```python
from build123d import *

# Parameters (mm, degrees)
SKETCH1_W           = 135.25
SKETCH1_H           = 90
BOSS_EXTRUDE1_DEPTH = 22
SKETCH4_W           = 5
SKETCH4_H           = 19
CUT_EXTRUDE1_DEPTH  = 91
SKETCH5_W           = 117.25
SKETCH5_H           = 11
CUT_EXTRUDE2_DEPTH  = 91
FILLET1_R           = 10
FILLET2_R           = 10
FILLET3_R           = 10
FILLET4_R           = 10
FILLET5_R           = 10
SKETCH6_R           = 4
CUT_EXTRUDE3_DEPTH  = 136.25


with BuildPart() as part:
    # Sketch1 → Boss-Extrude1 (new body)
    with BuildSketch(Plane(origin=(0, 0, 0), x_dir=(1, 0, 0), z_dir=(0, 1, 0))):
        Rectangle(SKETCH1_W, SKETCH1_H)
    extrude(amount=BOSS_EXTRUDE1_DEPTH)

    # Sketch4 → Cut-Extrude1 (cut, through all)
    with BuildSketch(Plane.XY.offset(45)):
        with Locations((-61.125, 9.5)):
            Rectangle(SKETCH4_W, SKETCH4_H)
        with Locations((61.125, 9.5)):
            Rectangle(SKETCH4_W, SKETCH4_H)
    extrude(amount=-CUT_EXTRUDE1_DEPTH, mode=Mode.SUBTRACT)

    # Sketch5 → Cut-Extrude2 (cut, through all)
    with BuildSketch(Plane(origin=(0, 0, -45), x_dir=(-1, 0, 0), z_dir=(0, 0, -1))):
        Rectangle(SKETCH5_W, SKETCH5_H)
    extrude(amount=-CUT_EXTRUDE2_DEPTH, mode=Mode.SUBTRACT)

    # Fillet1
    fillet1_edges = [part.edges().sort_by_distance(p)[0] for p in [
        (0, 5.5, 45),
    ]]
    fillet(fillet1_edges, radius=FILLET1_R)

    # Fillet2
    fillet2_edges = [part.edges().sort_by_distance(p)[0] for p in [
        (-65.625, 0, 45),
    ]]
    fillet(fillet2_edges, radius=FILLET2_R)

    # Fillet3
    fillet3_edges = [part.edges().sort_by_distance(p)[0] for p in [
        (65.625, 0, 45),
    ]]
    fillet(fillet3_edges, radius=FILLET3_R)

    # Fillet4
    fillet4_edges = [part.edges().sort_by_distance(p)[0] for p in [
        (-65.625, 0, -45),
    ]]
    fillet(fillet4_edges, radius=FILLET4_R)

    # Fillet5
    fillet5_edges = [part.edges().sort_by_distance(p)[0] for p in [
        (65.625, 0, -45),
    ]]
    fillet(fillet5_edges, radius=FILLET5_R)

    # Sketch6 → Cut-Extrude3 (cut, through all)
    with BuildSketch(Plane.ZY.offset(67.625)):
        with Locations((-38, 13)):
            Circle(SKETCH6_R)
    extrude(amount=-CUT_EXTRUDE3_DEPTH, mode=Mode.SUBTRACT)


solid = part.part
```
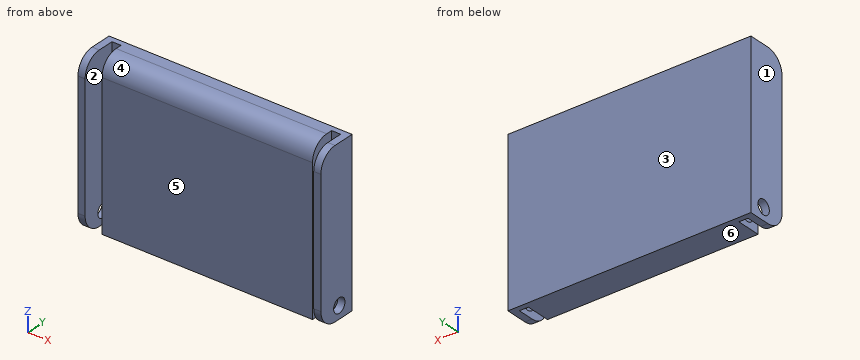
For this review, take the finished solid that the model builds, in its own axes (mm). Face numbers are marked on the shaded views. A direction names the side the tool comes from. Round coordinates to 2 decimals unless told otherwise and drop trailing zeros. Write each loop counter-clockwise with the first axis right and the second up, starting at its lowest first coordinate (ties: lowest second). Pieces come first, ordered by that corner, then holes. Notation, with made-up numbers: (11, 80.25) -> (42, 80.25) arc R23 ccw to (42, 98.25) -> close; hole circle Ø3 at (-17, 71). An arc over 180 degrees is marked (long way). Use one line per item in the form item = value.
Q1. The part is to be moulded in two halves that separate along X. For the marked faces 1, 2, 3 and 4, say which applies: released by +X, released by -X, zero draft, split by the parting line, or undercut.
Resolved:
face_1 = released by -X
face_2 = undercut
face_3 = zero draft
face_4 = undercut
Q2. Machinability: for the marked faces 5 and 6, which of the approach directions +Z, -Z, +X, -X, +Y, -Y give a long, thin tool a straight path to every point of the face, cutting with its end or side? Answer none if there is none.
Resolved:
face_5 = +Z, -Z, -Y
face_6 = -Z, +X, -X, +Y, -Y
Q3. Consider section B-B (x = 46). State the section outline as (y, z) points.
Resolved:
outline = (5.5, -45) -> (22, -45) -> (22, 45) -> (15.5, 45) arc R10 ccw to (5.5, 35) -> close; hole circle Ø8 at (13, -38)
Q4. Consider section D-D (z = -38). State the section outline as (x, y) points (3 decimals).
Resolved:
outline = (-67.625, 0.461) -> (-63.625, 0.461) -> (-63.625, 9) -> (-67.625, 9) -> close; (-67.625, 17) -> (-63.625, 17) -> (-63.625, 19) -> (-58.625, 19) -> (-58.625, 17) -> (58.625, 17) -> (58.625, 19) -> (63.625, 19) -> (63.625, 17) -> (67.625, 17) -> (67.625, 22) -> (-67.625, 22) -> close; (-58.625, 5.5) -> (58.625, 5.5) -> (58.625, 9) -> (-58.625, 9) -> close; (63.625, 0.461) -> (67.625, 0.461) -> (67.625, 9) -> (63.625, 9) -> close
Q5. Consider section C-C (y = 13). State the section outline as (x, z) points (3 decimals), then the cut area to 3 significant figures.
Resolved:
outline = (-67.625, -45) -> (-63.625, -45) -> (-63.625, -42) -> (-67.625, -42) -> close; (-67.625, -34) -> (-63.625, -34) -> (-63.625, 45) -> (-67.625, 45) -> close; (-58.625, -45) -> (58.625, -45) -> (58.625, -42) -> (-58.625, -42) -> close; (-58.625, -34) -> (58.625, -34) -> (58.625, 44.682) -> (-58.625, 44.682) -> close; (63.625, -45) -> (67.625, -45) -> (67.625, -42) -> (63.625, -42) -> close; (63.625, -34) -> (67.625, -34) -> (67.625, 45) -> (63.625, 45) -> close
area = 10,200 mm²
Q6. To check wall thickness, follow probe 1 along X at (y, z) = (6.25, -5) (3 decimals); probe 2 along Y at (x, z) = (25, -38); probe 3 along X at (y, z) = (3.25, 26.5) (3 decimals). State the ranges of each line that lie inside material, in increasing order. Write a range as from..to.
Resolved:
probe_1 = -67.625..-63.625, -58.625..58.625, 63.625..67.625
probe_2 = 5.5..9, 17..22
probe_3 = -67.625..-63.625, 63.625..67.625
Q7. Clearance check with flat-ended pins moving along their axes: pin 1 Ø5.5 at (x, z) = (60.5, 7) entering from -Y; pin 2 Ø3 at (x, y) = (15.5, 6) entering from +Z. State where each tip first meets the part, or that it passes through.
Resolved:
pin_1 = 5.5
pin_2 = 41
Q8. Consider section A-A (z = -20). State the section outline as (x, y) points (3 decimals), then the cut area to 3 significant figures.
Resolved:
outline = (-67.625, 0) -> (-63.625, 0) -> (-63.625, 19) -> (-58.625, 19) -> (-58.625, 5.5) -> (58.625, 5.5) -> (58.625, 19) -> (63.625, 19) -> (63.625, 0) -> (67.625, 0) -> (67.625, 22) -> (-67.625, 22) -> close
area = 2,140 mm²
